Autodesk Inventor part; units mm, degrees
ref_plane "YZ Plane" through (0, 0, 0) normal (1, 0, 0) x (0, 1, 0)
ref_plane "XZ Plane" through (0, 0, 0) normal (0, 1, 0) x (-1, 0, 0)
ref_plane "XY Plane" through (0, 0, 0) normal (0, 0, 1) x (1, 0, 0)
sketch "Sketch1" plane through (0, 0, 0) normal (0, 1, 0) x (-1, 0, 0)
  arc A0 (92.5, 31.0634) -> (-57.5, 31.0634) centre (17.5, -259.4104) ccw
  arc A1 (82.5, -7.6665) -> (92.5, 31.0634) centre (87.5, 11.6984) ccw
  arc A2 (-57.5, 31.0634) -> (-47.5, -7.6665) centre (-52.5, 11.6984) ccw
  arc A3 (82.5, -7.6665) -> (-47.5, -7.6665) centre (17.5, -259.4104) ccw
  line L0 (35, 0) -> (0, 0)
  line L1 (0, 0) -> (0, -50)
  line L2 (0, -50) -> (35, -50)
  line L3 (35, -50) -> (35, 0)
  point P0 (40, -0.7704)
  dimension "d0" = 140
  dimension "d1" = 20
  dimension "d2" = 52.5
  dimension "d4" = 300
  dimension "d5" = 50
  dimension "d8" = 35
  dimension "d9" = 52.5
extrude "Extrusion1" add sketch "Sketch1" along normal blind 4
sketch "Sketch2" plane through (0, 4, 0) normal (0, 1, 0) x (1, 0, 0)
  line L0 (0, 30) -> (-3, 30)
  line L1 (-3, 30) -> (-3, 20)
  line L2 (-3, 20) -> (0, 20)
  line L3 (0, 20) -> (0, 30)
  line L4 (-35, 30) -> (-32, 30)
  line L5 (-32, 30) -> (-32, 20)
  line L6 (-32, 20) -> (-35, 20)
  line L7 (-35, 20) -> (-35, 30)
  line L8 (0, 0) -> (0, 50)
  line L9 (-35, 50) -> (-35, 0)
  point P0 (-35, 25)
  dimension "d10" = 3
  dimension "d11" = 3
  dimension "d12" = 10
extrude "Extrusion2" add sketch "Sketch2" along normal blind 10
sketch "Sketch3" plane through (0, 4, 0) normal (0, 1, 0) x (1, 0, 0)
  line L0 (-35, 15) -> (0, 15)
  line L1 (0, 15) -> (0, 8)
  line L2 (0, 8) -> (-35, 8)
  line L3 (-35, 8) -> (-35, 15)
  line L4 (0, 0) -> (0, 20)
  line L5 (-35, 20) -> (-35, 0)
  line L6 (-35, 50) -> (-35, 0)
  point P0 (-35, 25)
  dimension "d15" = 7
  dimension "d16" = 10
extrude "Extrusion3" add sketch "Sketch3" along normal blind 8
sketch "Sketch4" plane through (0, 0, 0) normal (1, 0, 0) x (0, 0, -1)
  circle A0 centre (25, 9) radius 1.375
  line L0 (30, 4) -> (30, 14)
  line L1 (20, 14) -> (30, 14)
  point P0 (0, 0)
  point P1 (30, 9)
  point P2 (25, 14)
  dimension "d19" = 2.75
extrude "Extrusion4" cut sketch "Sketch4" against normal through all
sketch "Sketch5" plane through (0, 4, 0) normal (0, 1, 0) x (1, 0, 0)
  line L0 (-25, 37.5) -> (-10, 37.5)
  line L1 (-10, 37.5) -> (-10, 41.5)
  line L2 (-10, 41.5) -> (-25, 41.5)
  line L3 (-25, 41.5) -> (-25, 37.5)
  line L4 (0, 20) -> (0, 30)
  line L5 (-35, 50) -> (-35, 30)
  line L6 (0, 30) -> (0, 50)
  point P0 (0, 0)
  point P1 (-10, 39.5)
  point P2 (0, 25)
  dimension "d22" = 4
  dimension "d23" = 15
  dimension "d26" = 14.5
  dimension "d27" = 10
  dimension "d28" = 10
extrude "Extrusion5" add sketch "Sketch5" along normal blind 3.625
chamfer "Chamfer1" distance 2 angle 45 12 edges at (-17.5, 4, -15) (-32, 4, -25) (-33.5, 4, -30) (-33.5, 4, -20) (-17.5, 4, -8) (-3, 4, -25) (-1.5, 4, -30) (-1.5, 4, -20) (-10, 4, -39.5) (-17.5, 4, -41.5) (-17.5, 4, -37.5) (-25, 4, -39.5)
sketch "Sketch6" plane through (0, 4, 0) normal (0, 1, 0) x (1, 0, 0)
  circle A0 centre (-17.5, 81.5) radius 42
  line L0 (0, 0) -> (0, 50)
  line L1 (0, 50) -> (-35, 50)
  point P0 (0, 25)
  point P1 (-17.5, 50)
  dimension "d32" = 56.5
  dimension "d33" = 84
extrude "Extrusion6" cut sketch "Sketch6" along normal through all both and the other way through all
equation "\"d2\" = d9"
equation "\"d11\" = d10"
equation "\"d27\" = d28"
properties part number "paddle"
For this review, take the finished solid that the model builds, in its own axes (mm). A direction names the side the tool comes from. Coordinates: 2 decimals unless noted, no trailing zeros. Order: outer loops, then holes, each group sorted by start corner. A loop starts at its lowest first (then second) coordinate and runs counter-clockwise, first axis right, second up. Notation, with made-up numbers: (66.5, -20) - (70.5, -20) arc R34 ccw to (70.5, 12) - close; hole circle Ø5 at (50, 66.25). An arc over 180 degrees is marked (long way). Answer as CSV lines item,"result". Start each with the question number.
1) Machinability: for faces 1 (the flat face through (-18, 9, -15)), 2 (the cylindrical face through (24.261, 1.972, -2.786)), 3 (the flat face through (-34, 10, -30)), 4 (the flat face through (-32, 11, -25)), which of the approach directions +Z, -Z, +X, -X, +Y, -Y give a long, thin tool a straight path to every point of the face, cutting with its end or side? Answer none if there is none.
2) Add section A-A (z = 13.5). State the section outline as (x, y) points.
3) Add section B-B (x = 38). State the section outline as (y, z) points.
4) To check wall thickness, follow line 1 along Y through (x, z) = (-0.9, -25) (3 decimals); line 2 along X through (y, z) = (7, -26); line 3 along Z through (x, y) = (-27, 8.5). State the ranges of each line that lie inside material, in increasing order. Write a range as [from, to].
5) Insertion check: P1, Ø1, axis at y = 4.5, z = -27.5, coming from the +X side; P2, Ø6, axis at y = 5.5, z = -8.5, coming from the +X side; P3, Ø3.5, axis at x = -17, z = -11, coming from the +Y side. Each pin has a flat end and moves straight along its axis. Give the tip position at first contact, or say it passes through.
6) Draft analysis for pull direction Z (two halves, no side actions). For faces 5 (the flat face through (-34, 14, -25)), 6 (the flat face through (-1, 10, -30)), 7 (the flat face through (-17, 4, -27)), state which applies: +Z half, -Z half, draft (parallel to the pull), parting line (faces both ways), or undercut.
Result:
1,face 1,"+X, -X, +Y"
1,face 2,"-Z, +Y, -Y"
1,face 3,"-Z, +X, -X, +Y"
1,face 4,"-Z, +Y"
2,outline,"(-107.42, 0) - (72.42, 0) - (72.42, 4) - (-107.42, 4) - close"
3,outline,"(0, -5.4) - (4, -5.4) - (4, 35.41) - (0, 35.41) - close"
4,line 1,"[0, 7.625], [10.375, 14]"
4,line 2,"[-35, -32], [-3, 0]"
4,line 3,"[-15, -8]"
5,P1,"x = 0"
5,P2,"x = 62"
5,P3,"y = 12"
6,face 5,"draft"
6,face 6,"-Z half"
6,face 7,"undercut"
